The listing builds one solid part. Answer for the finished solid, in the listing's coordinates (mm). Give positions to 0.01 mm unless a question says otherwise; leave off trailing zeros. Loops run counter-clockwise (first coordinate to the right, second up) from the corner with the lowest first, then second, coordinate; pieces in that order, holes last. Notation, with made-up numbers: M -5,-24.5 L 15,-24.5 A15 cw 15,-20.5 Z; hole C 47.25,8 d7. An arc over 180 degrees is marked long. One line per item, written item: value. Start each with the question number.
Q1. Consider L1, parallel to Y at x = 0.35, z = -76.5; L2, parallel to Z at x = 0.4, y = 3.5; L3, parallel to Y at x = -1.4, z = -89.5. Determine where each line is inside the solid, lowest interval first.
Q2. A cutting plane is placed at A-A, the plane z = -82.5. Determine the outline of the cut face in (x, y).
Q3. Flat-ended cylindrical pins translate along their axes: pin 1 (2.5 mm diameter, centred on y = -3, z = -38.5, fed in from -X); pin 2 (1 mm diameter, centred on x = 0.5, y = -2, fed in from +Z); pin 3 (1.5 mm diameter, centred on y = -2, z = -34, fed in from +X). Find the tip coordinate at first contact, or state that the pin passes through.
Q4. A cutting plane is placed at B-B, the plane z = -130.5. Determine the outline of the cut face in (x, y).
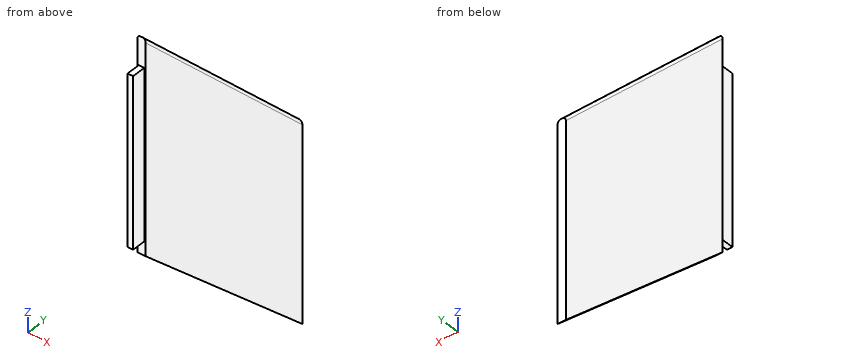
from build123d import *

# Parameters (mm, degrees)
EXTRUDE_1_DEPTH      = 1.5
EXTRUDE_1_DEPTH_BACK = 1.5
EXTRUDE_2_DEPTH      = 1
EXTRUDE_2_DEPTH_BACK = 1
SKETCH_1_3_W         = 61.5
SKETCH_1_3_H         = 5
FILLET_START         = -1
FILLET_1_DEPTH       = 102


with BuildPart() as part:
    # Sketch 1 → Extrude 1 (new, two sides: drawn at the far end of the back side and taken through both)
    with BuildSketch(Plane(origin=(0, 0, 0), x_dir=(0, 0, -1), z_dir=(1, 0, 0)).offset(-EXTRUDE_1_DEPTH_BACK)):
        Polygon((142, 70), (70, 70), (0, 0), (77, 0), align=None)
    extrude(amount=EXTRUDE_1_DEPTH + EXTRUDE_1_DEPTH_BACK)

    # Sketch 1_3 → Extrude 2 (add, two sides: drawn at the far end of the back side and taken through both)
    with BuildSketch(Plane(origin=(0, 0, 0), x_dir=(0, 0, -1), z_dir=(1, 0, 0)).offset(-EXTRUDE_2_DEPTH_BACK)):
        with Locations((41.25, -2.5)):
            Rectangle(SKETCH_1_3_W, SKETCH_1_3_H)
    extrude(amount=EXTRUDE_2_DEPTH + EXTRUDE_2_DEPTH_BACK)

    # Fillet 1: read off the stored shape, not the designer's step
    # Fillet 1 outline → Fillet 1 (cut)
    with BuildSketch(Plane(origin=(0, 0, 0), x_dir=(1, 0, 0), z_dir=(0, 0.7071067811865476, -0.7071067811865474)).offset(FILLET_START)):
        with BuildLine():
            Line((-1.5, 0), (-0.5, 0))
            add(Edge.make_bspline(
                [(-0.5, 0), (-1.5, 0), (-1.5, 1)],
                knots=[0, 0, 0, 1, 1, 1], degree=2, weights=[1, 0.707106781, 1]))
            Line((-1.5, 1), (-1.5, 0))
        make_face()
        with BuildLine():
            add(Edge.make_bspline(
                [(1.5, 1), (1.5, 0), (0.5, 0)],
                knots=[0, 0, 0, 1, 1, 1], degree=2, weights=[1, 0.707106781, 1]))
            Line((0.5, 0), (1.5, 0))
            Line((1.5, 0), (1.5, 1))
        make_face()
    extrude(amount=FILLET_1_DEPTH, mode=Mode.SUBTRACT)


solid = part.part
Answer block:
1. L1: 0 to 70
1. L2: -80.25 to -3.5
1. L3: 13.46 to 70
2. outline: M -1.5,5.92 L 1.5,5.92 L 1.5,70 L -1.5,70 Z
3. pin 1: x = -1
3. pin 2: z = -10.5
3. pin 3: x = 1
4. outline: M -1.5,57.62 L 1.5,57.62 L 1.5,70 L -1.5,70 Z
